Verification items for the finished model (mm, model axes). Coordinates: 2 decimals unless noted, no trailing zeros. Loops run counter-clockwise (first coordinate to the right, second up) from the corner with the lowest first, then second, coordinate; pieces in that order, holes last. Notation, with made-up numbers: (31, 55.5) -> (70, 55.5) arc R20 ccw to (70, 72.5) -> close; hole circle Ø4 at (-6, 17.5). An arc over 180 degrees is marked (long way). Answer as a JSON object with one key per item and string values. Group by question number.
Q1. Cross-section at A-A on y = -1.2. Record the boundary of the cut face in (x, z).
Q2. Cross-section at C-C on z = 2.3. Record the boundary of the cut face in (x, y), and give its area (3 significant figures).
Q3. Gauge pin test, flat ends, axial feed: pin 1 Ø3.5 at (x, z) = (-11.8, 0) entering from -Y; pin 2 Ø1.8 at (x, z) = (-2, 0) entering from -Y. Record the tip position at first contact, or that the pin passes through.
Q4. Release check for a two-part mould opening along X. For faces 1 (the cylindrical face through (-0.158, 1.521, 1.787)), 2 (the flat face through (0, 3, 0)) record: released by +X, released by -X, zero draft, split by the parting line, or undercut.
Q5. Cross-section at D-D on x = 9.75. Record the boundary of the cut face in (y, z), and give its area (3 significant figures).
Q6. Cross-section at B-B on y = 1.3. Record the boundary of the cut face in (x, z), and give its area (3 significant figures).
Q7. Scan lines: L1, parallel to X at y = 1, z = 0; L2, parallel to X at y = 1, z = 0.45; L3, parallel to Y at x = 6.5, z = -0.65. Record each from-to range of solid material in increasing order.
```python
from build123d import *
from build123d.topology import SkipClean

# Parameters (mm, degrees)
SKETCH1_R           = 1.5
BOSS_EXTRUDE1_DEPTH = 3
SKETCH2_OUTSIDE_W   = 37.67
SKETCH2_OUTSIDE_H   = 14.07
CUT_EXTRUDE1_DEPTH  = 16.396103403
BOSS_EXTRUDE2_START = -3
SKETCH3_R           = 1.5
BOSS_EXTRUDE2_DEPTH = 2


with BuildPart() as part:
    # Sketch1 → Boss-Extrude1 (new body)
    with BuildSketch(Plane(origin=(0, 0, 0), x_dir=(1, 0, 0), z_dir=(0, 1, 0))):
        with BuildLine():
            Line((-11.8, 3), (11.8, 3))
            ThreePointArc((11.8, 3), (14.8, 0), (11.8, -3))
            Line((11.8, -3), (-11.8, -3))
            ThreePointArc((-11.8, -3), (-14.8, 0), (-11.8, 3))
        make_face()
        with Locations(Location((-11.8, 0, 0), (0, 0, 270))):
            Circle(SKETCH1_R, mode=Mode.SUBTRACT)
        with Locations(Location((11.8, 0, 0), (0, 0, 270))):
            Circle(SKETCH1_R, mode=Mode.SUBTRACT)
    extrude(amount=BOSS_EXTRUDE1_DEPTH)

    # Sketch2 outside → Cut-Extrude1 (cut, through all)
    with SkipClean():  # the faces are left unmerged after this step: merging them gives an invalid solid
        with BuildSketch(Plane(origin=(0, 3, 0), x_dir=(1, 0, 0), z_dir=(0, 1, 0))):
            Rectangle(SKETCH2_OUTSIDE_W, SKETCH2_OUTSIDE_H)
            with BuildLine():
                ThreePointArc((-11.189655172, 2.937257086), (-14.8, 0), (-11.189655172, -2.937257086))
                ThreePointArc((-11.189655172, -2.937257086), (0, -1.786970337), (11.189655172, -2.937257086))
                ThreePointArc((11.189655172, -2.937257086), (14.8, 0), (11.189655172, 2.937257086))
                ThreePointArc((11.189655172, 2.937257086), (0, 1.786970337), (-11.189655172, 2.937257086))
            make_face(mode=Mode.SUBTRACT)
        extrude(amount=-CUT_EXTRUDE1_DEPTH, mode=Mode.SUBTRACT)

    # Sketch3 → Boss-Extrude2 (add)
    # profile 1 of 2: a face of its own
    with SkipClean():  # the faces are left unmerged after this step: merging them gives an invalid solid
        with BuildSketch(Plane(origin=(0, 3, 0), x_dir=(1, 0, 0), z_dir=(0, 1, 0)).offset(BOSS_EXTRUDE2_START)):
            with BuildLine():
                ThreePointArc((-11.189655172, -2.937257086), (-9.472873609, -1.893273028), (-8.8, 0))
                ThreePointArc((-8.8, 0), (-9.472873609, 1.893273028), (-11.189655172, 2.937257086))
                ThreePointArc((-11.189655172, 2.937257086), (-14.8, 0), (-11.189655172, -2.937257086))
            make_face()
            with Locations(Location((-11.8, 0, 0), (0, 0, 270))):
                Circle(SKETCH3_R, mode=Mode.SUBTRACT)
        # profile 2 of 2: a face of its own
        with BuildSketch(Plane(origin=(0, 3, 0), x_dir=(1, 0, 0), z_dir=(0, 1, 0)).offset(BOSS_EXTRUDE2_START)):
            with BuildLine():
                ThreePointArc((11.189655172, -2.937257086), (13.693273028, -2.327126391), (14.8, 0))
                ThreePointArc((14.8, 0), (13.693273028, 2.327126391), (11.189655172, 2.937257086))
                ThreePointArc((11.189655172, 2.937257086), (8.8, 0), (11.189655172, -2.937257086))
            make_face()
            with Locations(Location((11.8, 0, 0), (0, 0, 270))):
                Circle(SKETCH3_R, mode=Mode.SUBTRACT)
        extrude(amount=-BOSS_EXTRUDE2_DEPTH)


solid = part.part
```
Computed values:
{
 "1": {"outline": "circle Ø6 at (-11.8, 0); circle Ø6 at (11.8, 0); hole circle Ø3 at (-11.8, 0); hole circle Ø3 at (11.8, 0)"},
 "2": {"outline": "(-13.73, -2) -> (-9.87, -2) -> (-9.87, 0) -> (-7.49, 0) -> (-7.49, 3) -> (-13.73, 3) -> close; (7.49, 0) -> (9.87, 0) -> (9.87, -2) -> (13.73, -2) -> (13.73, 3) -> (7.49, 3) -> close", "area": "52.8 mm²"},
 "3": {"pin 1": "stops at y = -2", "pin 2": "stops at y = 0"},
 "4": {"face 1": "undercut", "face 2": "zero draft"},
 "5": {"outline": "(-2, -2.19) -> (0, -2.19) -> (0, -2.66) -> (3, -2.66) -> (3, 2.66) -> (0, 2.66) -> (0, 2.19) -> (-2, 2.19) -> close", "area": "24.7 mm²"},
 "6": {"outline": "(-11.19, -2.94) arc R55 cw to (11.19, -2.94) arc R3 ccw (long way) to (11.19, 2.94) arc R55 cw to (-11.19, 2.94) arc R3 ccw (long way) to start; hole circle Ø3 at (-11.8, 0); hole circle Ø3 at (11.8, 0)", "area": "118 mm²"},
 "7": {"L1": "x = -14.8 to -13.3, -10.3 to 10.3, 13.3 to 14.8", "L2": "x = -14.77 to -13.23, -10.37 to 10.37, 13.23 to 14.77", "L3": "y = 0 to 3"}
}
